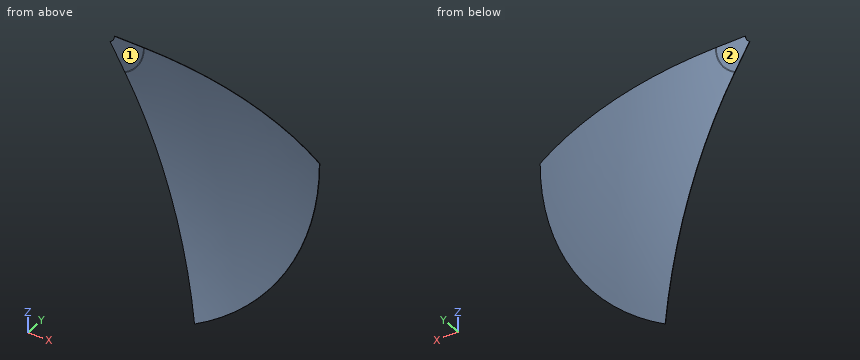
```python
from build123d import *

# Parameters (mm, degrees)
REVOLVE1_ANGLE = 60


with BuildPart() as part:
    # Sketch1 → Revolve1 (revolve)
    with BuildSketch(Plane.XY):
        with BuildLine():
            Line((10, -0.5), (45, -0.5))
            ThreePointArc((45, -0.5), (45.500946005, -0.500236893), (46.001891561, -0.50094757))
            ThreePointArc((46.001891561, -0.50094757), (176.838494864, -17.170276226), (299.5, -65.649534053))
            Line((299.5, -65.649534053), (299.740246695, -65.211034879))
            ThreePointArc((299.740246695, -65.211034879), (176.962949727, -16.686012882), (46.002837341, -0.000948465))
            ThreePointArc((46.002837341, -0.000948465), (45.501418895, -0.000237116), (45, 0))
            Line((45, 0), (10, 0))
            Line((10, 0), (10, -0.5))
        make_face()
    revolve(axis=Axis((0, -1000, 0), (0, 1, 0)), revolution_arc=REVOLVE1_ANGLE)


solid = part.part
```
Geometry: final body of the model. Coordinates: model frame, mm. Face numbers are marked on the shaded views. A direction names the side the tool comes from. Coordinates: 2 decimals unless noted, no trailing zeros. Answer in a Markdown table with one row per item. Add a question column.
Q1. Line query: L1, parallel to X at y = -54.5, z = -103.5; L2, parallel to Y at x = 74.5, z = -61.5; L3, parallel to Y at x = 139, z = -217.5. Output: solid intervals per line, ascending.
Q2. Contact query for flat-ended pins moving along their axis: P1, Ø1, axis at x = 262.5, z = -76, coming from the +Y side; P2, Ø4, axis at x = 256, z = -66.5, coming from the +Y side; P3, Ø12, axis at x = 47, z = -30.5, coming from the +Y side. Output: stop coordinate, or through.
Q3. Reachability of the marked faces 1 and 2 from +Z, -Z, +X, -X, +Y, -Y: full face, straight path, thin tool, end or side. Return the list, or none.
Completed:
| question | item | result |
|---|---|---|
| 1 | L1 | x = 258.01 to 259.23 |
| 1 | L2 | y = -3.02 to -2.52 |
| 1 | L3 | y = -45.27 to -44.72 |
| 2 | P1 | stops at y = -51.43 |
| 2 | P2 | stops at y = -46.67 |
| 2 | P3 | stops at y = -0.02 |
| 3 | face 1 | +Z, -X, -Y |
| 3 | face 2 | +Z, -Z, +X, -X, +Y |
